Geometry: final body of the model. Coordinates: model frame, mm. Face numbers are marked on the shaded views. A direction names the side the tool comes from. Give positions to 0.01 mm unless a question says otherwise; leave off trailing zeros. Write each loop counter-clockwise with the first axis right and the second up, starting at its lowest first coordinate (ties: lowest second). Pieces come first, ordered by that corner, then holes. Notation, with made-up numbers: (23.5, 79.25) -> (77.5, 79.25) arc R19 ccw to (77.5, 114.25) -> close; hole circle Ø7 at (-16.5, 71). An arc over 180 degrees is marked (long way). Answer as a JSON object with one key per item and string values.
from build123d import *

# Parameters (mm, degrees)
CROQUIS1_R                 = 17.5
SALIENTE_EXTRUIR1_DEPTH    = 20
CROQUIS2_R                 = 9.125
CROQUIS2_R_2               = 4.125
SALIENTE_EXTRUIR2_DEPTH    = 10
CORTAR_EXTRUIR1_START      = -20
CROQUIS3_R                 = 19
CORTAR_EXTRUIR1_DEPTH      = 20
CORTAR_EXTRUIR2_DEPTH      = 32.674365543
CORTAR_EXTRUIR2_DEPTH_BACK = 32.674365543
CROQUIS4_R                 = 2.05
CROQUIS5_R                 = 4.125
CORTAR_EXTRUIR3_DEPTH      = 32.674365543


with BuildPart() as part:
    # Croquis1 → Saliente-Extruir1 (new body)
    with BuildSketch(Plane.XY):
        Circle(CROQUIS1_R)
    extrude(amount=SALIENTE_EXTRUIR1_DEPTH)

    # Croquis2 → Saliente-Extruir2 (add)
    with BuildSketch(Plane(origin=(0, 0, 0), x_dir=(-1, 0, 0), z_dir=(0, 0, -1))):
        with Locations(Location((0, 0, 0), (0, 0, 180))):
            Circle(CROQUIS2_R)
        Circle(CROQUIS2_R_2, mode=Mode.SUBTRACT)
    extrude(amount=SALIENTE_EXTRUIR2_DEPTH)

    # Croquis3 → Cortar-Extruir1 (cut)
    with BuildSketch(Plane.XY.offset(20).offset(CORTAR_EXTRUIR1_START)):
        Circle(CROQUIS3_R)
        Polygon((0, 17.5), (2.778370843, 15.756924048), (5.985352508, 16.444620864), (8, 13.856406461), (11.24878317, 13.405777755), (12.25671109, 10.284601755), (15.155444566, 8.75), (15.035081933, 5.472322293), (17.234135678, 3.038843109), (16, 0), (17.234135678, -3.038843109), (15.035081933, -5.472322293), (15.155444566, -8.75), (12.25671109, -10.284601755), (11.24878317, -13.405777755), (8, -13.856406461), (5.985352508, -16.444620864), (2.778370843, -15.756924048), (0, -17.5), (-2.778370843, -15.756924048), (-5.985352508, -16.444620864), (-8, -13.856406461), (-11.24878317, -13.405777755), (-12.25671109, -10.284601755), (-15.155444566, -8.75), (-15.035081933, -5.472322293), (-17.234135678, -3.038843109), (-16, 0), (-17.234135678, 3.038843109), (-15.035081933, 5.472322293), (-15.155444566, 8.75), (-12.25671109, 10.284601755), (-11.24878317, 13.405777755), (-8, 13.856406461), (-5.985352508, 16.444620864), (-2.778370843, 15.756924048), align=None, mode=Mode.SUBTRACT)
    extrude(amount=CORTAR_EXTRUIR1_DEPTH, mode=Mode.SUBTRACT)

    # Croquis4 → Cortar-Extruir2 (cut, two sides: drawn at the far end of the back side and taken through both)
    with BuildSketch(Plane(origin=(0, 0, 0), x_dir=(1, 0, 0), z_dir=(0, 1, 0)).offset(-CORTAR_EXTRUIR2_DEPTH_BACK)):
        with Locations(Location((0, 5, 0), (0, 0, 270))):
            Circle(CROQUIS4_R)
    extrude(amount=CORTAR_EXTRUIR2_DEPTH + CORTAR_EXTRUIR2_DEPTH_BACK, mode=Mode.SUBTRACT)

    # Croquis5 → Cortar-Extruir3 (cut, through all)
    with BuildSketch(Plane(origin=(0, 0, 0), x_dir=(-1, 0, 0), z_dir=(0, 0, -1))):
        Circle(CROQUIS5_R)
    extrude(amount=-CORTAR_EXTRUIR3_DEPTH, mode=Mode.SUBTRACT)


solid = part.part
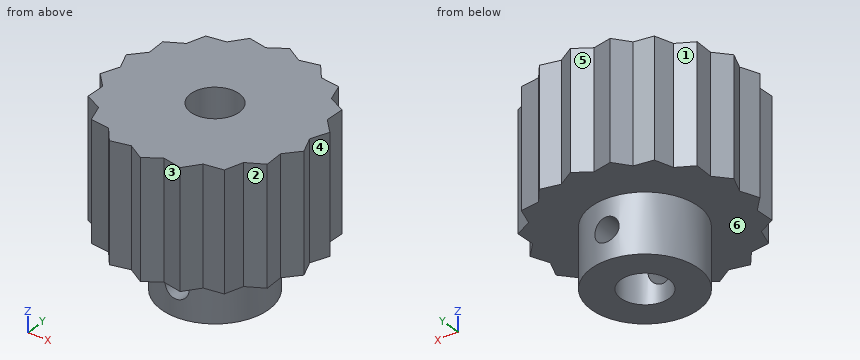
Q1. Cut plane D-D (x = -7.5). Return the cut outline in (y, z), and give its area (3 significant figures).
Values:
{"outline": "(-14.5, 0) -> (-5.2, 0) -> (-5.2, -10) -> (5.2, -10) -> (5.2, 0) -> (14.5, 0) -> (14.5, 20) -> (-14.5, 20) -> close", "area": "684 mm²"}
Q2. Cut plane C-C (z = -3.5). Return the cut outline in (x, y) (3 decimals).
Values:
{"outline": "(-1.397, -9.017) -> (-1.397, -3.881) arc R4.125 cw to (-1.397, 3.881) -> (-1.397, 9.017) arc R9.125 ccw to start; (1.397, -9.017) arc R9.125 ccw to (1.397, 9.017) -> (1.397, 3.881) arc R4.125 cw to (1.397, -3.881) -> close"}
Q3. Cut plane A-A (y = 1). Return the cut outline in (x, z), and give its area (3 significant figures).
Values:
{"outline": "(-16.41, 0) -> (-9.07, 0) -> (-9.07, -10) -> (-4, -10) -> (-4, 20) -> (-16.41, 20) -> close; (4, -10) -> (9.07, -10) -> (9.07, 0) -> (16.41, 0) -> (16.41, 20) -> (4, 20) -> close", "area": "598 mm²"}
Q4. Mould query, pull axis X, two halves, no side actions, for the marked faces 1, 2 and 3. Classes: pulls with the +X half, pulls with the -X half, needs draft (parallel to the pull), parting line crosses it, or undercut.
Values:
{"face 1": "pulls with the -X half", "face 2": "pulls with the +X half", "face 3": "undercut"}
Q5. Set-up query: the marked faces 4, 5 and 6. Return all of +Z, -Z, +X, -X, +Y, -Y with unobstructed straight access to the full face (end or side cutting, diameter ignored); none if empty.
Values:
{"face 4": "+Z, -Z, +X", "face 5": "+Z, -Z, +Y", "face 6": "-Z"}
Q6. Cut plane B-B (x = 3.5). Return the cut outline in (y, z), and give its area (3 significant figures).
Values:
{"outline": "(-15.91, 0) -> (-8.43, 0) -> (-8.43, -10) -> (-2.18, -10) -> (-2.18, 20) -> (-15.91, 20) -> close; (2.18, -10) -> (8.43, -10) -> (8.43, 0) -> (15.91, 0) -> (15.91, 20) -> (2.18, 20) -> close", "area": "674 mm²"}
Q7. First-contact query: P1, Ø2, axis at y = -5.5, z = 11, coming from the -X side; P2, Ø5, axis at x = 0, y = 0, coming from the -Z side; P3, Ø1.5, axis at x = 8.5, z = -5, coming from the -Y side; P4, Ø6, axis at x = 0.5, y = 2, coming from the +Z side. Flat tips, straight axial feed; report the tip coordinate or a pass-through.
Values:
{"P1": "x = -15.91", "P2": "through", "P3": "y = -4.82", "P4": "z = 20"}
Q8. Material intervals for L1, parallel to Z at x = 0, y = -5.3; L2, parallel to X at y = -8.5, z = 11.5; L3, parallel to Z at x = -2, y = 9, sorted ascending. Write a range as from..to.
Values:
{"L1": "-10..-7.05, -2.95..20", "L2": "-15.15..15.15", "L3": "0..20"}
